Verification items for the finished model (mm, model axes). A direction names the side the tool comes from. Coordinates: 2 decimals unless noted, no trailing zeros. Write each loop counter-clockwise with the first axis right and the second up, starting at its lowest first coordinate (ties: lowest second). Pieces come first, ordered by that corner, then holes. Notation, with made-up numbers: M -26.5,49 L 7.5,49 A35 cw 7.5,85 Z; hole C 64,83.25 d8. An arc over 180 degrees is marked long. One line per item, written item: value.
Autodesk Fusion 360 part; units mm, degrees
sketch "Sketch1" plane through (0, 0, 0) normal (0, 1, 0) x (1, 0, 0)
  line L0 (86, 73.5) -> (-86, 73.5)
  line L1 (-86, 73.5) -> (-86, -73.5)
  line L2 (-86, -73.5) -> (86, -73.5)
  line L3 (86, -73.5) -> (86, 73.5)
  line L4 (86, 73.5) -> (-86, -73.5) construction
  line L5 (-86, 73.5) -> (86, -73.5) construction
  line L6 (-77, -64.5) -> (77, -64.5)
  line L7 (77, -64.5) -> (77, 64.5)
  line L8 (77, 64.5) -> (-77, 64.5)
  line L9 (-77, 64.5) -> (-77, -64.5)
  line L10 (102, -89.5) -> (102, 89.5)
  line L11 (102, 89.5) -> (-102, 89.5)
  line L12 (-102, 89.5) -> (-102, -89.5)
  line L13 (-102, -89.5) -> (102, -89.5)
  dimension "d1" = 172
  dimension "d6" = 147
  dimension "d15" = 16
extrude "Extrude1" add sketch "Sketch1" along normal blind 9 contours L0 L1 L2 L3
ref_plane "WorkPlane1" through (0, 9, 0) normal (0, 1, 0) x (0, 0, 1)
sketch "Sketch2" plane through (0, 9, 0) normal (0, 1, 0) x (1, 0, 0)
  line L0 (-77, -64.5) -> (-77, 64.5)
  line L1 (-77, 64.5) -> (77, 64.5)
  line L2 (77, 64.5) -> (77, -64.5)
  line L3 (77, -64.5) -> (-77, -64.5)
  line L4 (86, -73.5) -> (86, 73.5)
  line L5 (86, 73.5) -> (-86, 73.5)
  line L6 (-86, 73.5) -> (-86, -73.5)
  line L7 (-86, -73.5) -> (86, -73.5)
  line L8 (95, -82.5) -> (95, 82.5)
  line L9 (95, 82.5) -> (-95, 82.5)
  line L10 (-95, 82.5) -> (-95, -82.5)
  line L11 (-95, -82.5) -> (95, -82.5)
  line L12 (-111, -98.5) -> (111, -98.5)
  line L13 (111, -98.5) -> (111, 98.5)
  line L14 (111, 98.5) -> (-111, 98.5)
  line L15 (-111, 98.5) -> (-111, -98.5)
  arc A0 (-56.3726, 98.5) -> (-111, 43.8726) centre (-56.3726, 43.8726) ccw
  arc A1 (-111, -43.8726) -> (-56.3726, -98.5) centre (-56.3726, -43.8726) ccw
  arc A2 (56.3726, -98.5) -> (111, -43.8726) centre (56.3726, -43.8726) ccw
  arc A3 (111, 43.8726) -> (56.3726, 98.5) centre (56.3726, 43.8726) ccw
  dimension "d11" = 9
  dimension "d16" = 25
extrude "Extrude2" add sketch "Sketch2" along normal blind 15 contours L0 L1 L2 L3 | L4 L5 L6 L7 | L8 L9 L10 L11 | L11 L12 A1 A2 | L9 L14 A0 A3
equation "d1 = CaseLength - 2 * SideWidth"
equation "CaseLength = 190 mm"
equation "CaseWidth = 165 mm"
equation "SideWidth = 9 mm"
equation "PanelHeight = 15 mm"
equation "d6 = CaseWidth - 2 * SideWidth"
equation "d8 = SideWidth"
equation "d10 = SideWidth"
equation "d11 = SideWidth"
equation "d12 = PanelHeight"
equation "FlangeWidth = 16 mm"
equation "d15 = FlangeWidth"
equation "d16 = SideWidth + FlangeWidth"
Item 1: Access from +Z, -Z, +X, -X, +Y, -Y to the whole of each face (thin tool, end or side, straight path). Record for faces 1 (the face through (-86, 4, -1)), 2 (the face through (86, 4, 1)), 3 (the face through (-1, 4, 73.5)), 4 (the face through (-77, 4, -1)).
The answers:
face 1: +Z, -Z, -X, -Y
face 2: +Z, -Z, +X, -Y
face 3: +Z, +X, -X, -Y
face 4: -Y
Item 2: Go/stop test with flat-tipped pins: P1, Ø2.5, axis at x = -39.5, y = 5.5, coming from the +Z side; P2, Ø2.5, axis at y = 6, z = 8, coming from the -X side; P3, Ø10, axis at x = -68.5, y = 19.5, coming from the +Z side. Record where each tip stops, or that it passes through.
The answers:
P1: stops at z = 73.5
P2: stops at x = -86
P3: stops at z = 98.03
Item 3: Cross-section at D-D, the plane y = 16.5. Enter the section's corners in (x, z).
The answers:
outline: M -95,-82.5 A54.63 ccw -56.37,-98.5 L 56.37,-98.5 A54.63 ccw 95,-82.5 L 95,82.5 A54.63 ccw 56.37,98.5 L -56.37,98.5 A54.63 ccw -95,82.5 Z
Item 4: Cross-section at A-A, the plane y = 4. Enter the section's corners in (x, z), and give its area (3 significant figures).
The answers:
outline: M -86,-73.5 L 86,-73.5 L 86,73.5 L -86,73.5 Z; hole M -77,-64.5 L 77,-64.5 L 77,64.5 L -77,64.5 Z
area: 5,420 mm²
Item 5: Draft check along Z on faces 5 (the face through (-1, 24, -1)), 6 (the face through (1, 4, -64.5)), 7 (the face through (1, 4, -73.5)). Enter one of: released by +Z, released by -Z, zero draft, split by the parting line, or undercut.
The answers:
face 5: zero draft
face 6: undercut
face 7: released by -Z
Item 6: Scan lines: line 1 (X direction, y = 7.5, z = 22.5); line 2 (Z direction, x = 21, y = 8); line 3 (Y direction, x = 70, z = -32.5). Record each from-to range of solid material in increasing order.
The answers:
line 1: x = -86 to -77, 77 to 86
line 2: z = -73.5 to -64.5, 64.5 to 73.5
line 3: y = 9 to 24
Item 7: Cross-section at B-B, the plane z = 71. Enter the section's corners in (x, y).
The answers:
outline: M -95,9 L -86,9 L -86,0 L 86,0 L 86,9 L 95,9 L 95,24 L -95,24 Z
Item 8: Cross-section at C-C, the plane x = -19.5. Enter the section's corners in (y, z).
The answers:
outline: M 0,-73.5 L 9,-73.5 L 9,-98.5 L 24,-98.5 L 24,98.5 L 9,98.5 L 9,73.5 L 0,73.5 L 0,64.5 L 9,64.5 L 9,-64.5 L 0,-64.5 Z
